Build history of the part. All positions in model axes, mm. Face numbers are marked on the shaded views. A direction names the side the tool comes from. Coordinates: 2 decimals unless noted, no trailing zeros. Write each loop counter-clockwise with the first axis right and the second up, starting at its lowest first coordinate (ties: lowest second). Pieces come first, ordered by that corner, then holes.
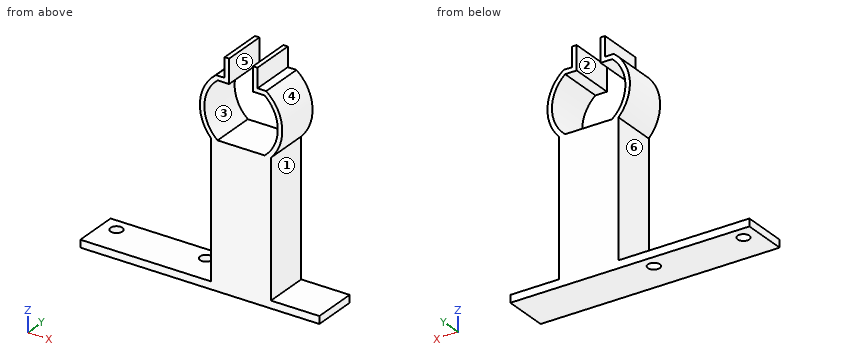
Autodesk Inventor part; units mm, degrees
ref_plane "YZ Plane" through (0, 0, 0) normal (1, 0, 0) x (0, 1, 0)
ref_plane "XZ Plane" through (0, 0, 0) normal (0, 1, 0) x (-1, 0, 0)
ref_plane "XY Plane" through (0, 0, 0) normal (0, 0, 1) x (1, 0, 0)
sketch "Sketch1" plane through (0, 0, 0) normal (0, 0, 1) x (1, 0, 0)
  circle A0 centre (-173.3589, -112.9) radius 2
  circle A1 centre (-143.3589, -112.9) radius 2
  circle A2 centre (-173.3589, -112.9) radius 2
  circle A3 centre (-143.3589, -112.9) radius 2
  line L0 (-178.3589, -108.4) -> (-98.3589, -108.4)
  line L1 (-98.3589, -108.4) -> (-98.3589, -123.4)
  line L2 (-98.3589, -123.4) -> (-178.3589, -123.4)
  line L3 (-178.3589, -123.4) -> (-178.3589, -108.4)
  point P0 (0, 0)
  dimension "d0" = 4
  dimension "d1" = 4
  dimension "d2" = 15
  dimension "d3" = 80
  dimension "d4" = 4.5
  dimension "d5" = 5
extrude "Extrusion1" add sketch "Sketch1" along normal blind 2.5
sketch "Sketch2" plane through (0, 0, 2.5) normal (0, 0, 1) x (1, 0, 0)
  line L0 (-178.3589, -123.4) -> (-98.3589, -123.4)
  line L1 (-98.3589, -123.4) -> (-98.3589, -108.4)
  line L2 (-98.3589, -108.4) -> (-178.3589, -108.4)
  line L3 (-178.3589, -108.4) -> (-178.3589, -123.4)
  circle A0 centre (-143.3589, -112.9) radius 2
  circle A1 centre (-173.3589, -112.9) radius 2
  line L4 (-122.2642, -87.4) -> (-126.8642, -87.4)
  line L5 (-124.5642, -87.4) -> (-124.5642, -147.4431) construction
  line L6 (-124.5642, -115.9) -> (-114.5642, -115.9) construction
  line L7 (-98.3589, -108.4) -> (-178.3589, -108.4)
  line L8 (-114.5642, -115.9) -> (-114.5642, -123.4)
  line L9 (-114.5642, -115.9) -> (-114.5642, -108.4)
  line L10 (-134.5642, -115.9) -> (-134.5642, -123.4)
  line L11 (-134.5642, -115.9) -> (-134.5642, -108.4)
  line L12 (-114.5642, -123.4) -> (-134.5642, -123.4)
  line L13 (-178.3589, -123.4) -> (-98.3589, -123.4)
  line L14 (-114.5642, -108.4) -> (-134.5642, -108.4)
  point P0 (0, 0)
  point P1 (-112.4142, -124.5353)
  point P2 (-112.4142, -107.2647)
  dimension "d8" = 10
extrude "Extrusion2" add sketch "Sketch2" along normal blind 45 contours L10 L11 L2 L9 L8 L0
sketch "Sketch3" plane through (-178.3589, -123.4, 0) normal (0, -1, 0) x (1, 0, 0)
  circle A0 centre (53.7947, 57.0153) radius 2.3 construction
  line L0 (53.7947, 57.0153) -> (53.7947, 47.7653) construction
  line L1 (53.7947, 57.0153) -> (65.8947, 57.0153) construction
  line L2 (53.7947, 47.7653) -> (61.5952, 47.7653) construction
  line L3 (53.7947, 47.7653) -> (45.9942, 47.7653) construction
  line L4 (53.7947, 66.2653) -> (61.5952, 66.2653) construction
  line L5 (53.7947, 66.2653) -> (45.9942, 66.2653) construction
  arc A1 (45.9942, 66.2653) -> (45.9942, 47.7653) centre (53.7947, 57.0153) ccw construction
  arc A2 (61.5952, 47.7653) -> (61.5952, 66.2653) centre (53.7947, 57.0153) ccw construction
  line L6 (61.6679, 66.4653) -> (53.9215, 66.4653)
  line L7 (53.9215, 66.4653) -> (45.9215, 66.4653)
  arc A3 (45.9215, 66.4653) -> (45.9215, 47.5653) centre (53.7947, 57.0153) ccw
  line L8 (45.9215, 47.5653) -> (53.7947, 47.5653)
  line L9 (53.7947, 47.5653) -> (61.6679, 47.5653)
  arc A4 (61.6679, 47.5653) -> (61.6679, 66.4653) centre (53.7947, 57.0153) ccw
  line L10 (62.1934, 67.9653) -> (59.2947, 67.9653)
  arc A5 (45.396, 67.9653) -> (45.396, 46.0653) centre (53.7947, 57.0153) ccw
  line L11 (45.396, 46.0653) -> (53.7947, 46.0653)
  line L12 (53.7947, 46.0653) -> (62.1934, 46.0653)
  arc A6 (62.1934, 46.0653) -> (62.1934, 67.9653) centre (53.7947, 57.0153) ccw
  line L13 (57.7947, 66.4653) -> (57.7947, 74.4653)
  line L14 (49.7947, 66.4653) -> (49.7947, 74.4653)
  line L15 (59.2947, 67.9653) -> (59.2947, 74.4653)
  line L16 (48.2947, 67.9653) -> (48.2947, 74.4653)
  line L17 (48.2947, 74.4653) -> (49.7947, 74.4653)
  line L18 (57.7947, 74.4653) -> (59.2947, 74.4653)
  line L19 (48.2947, 67.9653) -> (45.396, 67.9653)
  point P0 (178.3589, 0)
  dimension "d11" = 9.25
  dimension "d12" = 12.1
  dimension "d13" = 0.2
  dimension "d14" = 1.5
  dimension "d15" = 8
  dimension "d16" = 4
  dimension "d17" = 1.5
  dimension "d18" = 1.5
extrude "Extrusion3" add sketch "Sketch3" against normal blind 15 contours L6 L13 L18 L15 L10 A6 L12 L11 A5 L19 L16 L17 L14 L7 A3 L8 L9 A4
properties part number "sujetador_motor"
(1) Flat gauge pins, fed straight in: P1, Ø2.5, axis at y = -116.5, z = 70, coming from the -X side; P2, Ø0.9, axis at x = -118, y = -114.5, coming from the +Z side; P3, Ø4, axis at x = -148.5, y = -113.5, coming from the +Z side. Where does each tip first touch, or does it go through?
(2) Slice it at D-D, the plane x = -125.5. List the corners of the cut face in (y, z), and give its area (3 significant figures).
(3) Two-plate mould, pull along X, no slides. Class the marked faces 4, 5 and 6: pulls with the +X half, pulls with the -X half, needs draft (parallel to the pull), parting line crosses it, or undercut.
(4) Slice it at A-A, the plane y = -112.9. Give the number of separate pieces and of enclosed holes in the cut face, and give its area (3 significant figures).
(5) Slice it at B-B, the plane z = 57. List the corners of the cut face in (x, y), and give its area (3 significant figures).
(6) 3-axis set-ups, long thin cutter, end or side, ignore diameter. For the marked faces 1, 2 and 3: which of +Z, -Z, +X, -X, +Y, -Y reach the whole face in a straight line?
(7) Probe L1, parallel to X at y = -118.75, z = 71.5; L2, parallel to Z at x = -108, y = -117; L3, parallel to Z at x = -137, y = -123. List the from-to ranges inside material, lowest first.
Results:
1. P1: stops at x = -130.06
1. P2: stops at z = 67.97
1. P3: stops at z = 2.5
2. outline: (-123.4, 0) - (-108.4, 0) - (-108.4, 47.57) - (-123.4, 47.57) - close
2. area: 713 mm2
3. face 4: pulls with the +X half
3. face 5: undercut
3. face 6: pulls with the -X half
4. separate pieces: 3
4. enclosed holes: 0
4. area: 1,180 mm2
5. outline: (-138.36, -123.4) - (-136.86, -123.4) - (-136.86, -108.4) - (-138.36, -108.4) - close; (-112.26, -123.4) - (-110.76, -123.4) - (-110.76, -108.4) - (-112.26, -108.4) - close
5. area: 45.0 mm2
6. face 1: +X, +Y, -Y
6. face 2: +Z, +Y, -Y
6. face 3: +Y, -Y
7. L1: x = -130.06 to -128.56, -120.56 to -119.06
7. L2: z = 0 to 2.5
7. L3: z = 0 to 2.5, 51.03 to 63
